```python
from build123d import *

# Parameters (mm, degrees)
CROQUIS1_R              = 20
CROQUIS1_R_2            = 15
SALIENTE_EXTRUIR1_DEPTH = 10
CROQUIS2_R              = 20
SALIENTE_EXTRUIR2_DEPTH = 2
CROQUIS3_R              = 12.5
SALIENTE_EXTRUIR3_DEPTH = 30
CORTAR_EXTRUIR2_DEPTH   = 10


with BuildPart() as part:
    # Croquis1 → Saliente-Extruir1 (new body)
    with BuildSketch(Plane(origin=(0, 0, 0), x_dir=(1, 0, 0), z_dir=(0, 1, 0))):
        with Locations(Location((0, 0, 0), (0, 0, 270))):
            Circle(CROQUIS1_R)
        with Locations(Location((0, 0, 0), (0, 0, 270))):
            Circle(CROQUIS1_R_2, mode=Mode.SUBTRACT)
    extrude(amount=-SALIENTE_EXTRUIR1_DEPTH)

    # Croquis2 → Saliente-Extruir2 (add)
    with BuildSketch(Plane.XZ.offset(10)):
        with Locations(Location((0, 0, 0), (0, 0, 90))):
            Circle(CROQUIS2_R)
    extrude(amount=SALIENTE_EXTRUIR2_DEPTH)

    # Croquis3 → Saliente-Extruir3 (add)
    with BuildSketch(Plane.XZ.offset(12)):
        with Locations(Location((0, 0, 0), (0, 0, 270))):
            Circle(CROQUIS3_R)
    extrude(amount=SALIENTE_EXTRUIR3_DEPTH)

    # Croquis4 → Cortar-Extruir2 (cut, symmetric)
    with BuildSketch(Plane.XY):
        Polygon((-15.546090629, -15.510770255), (-15.546090629, -25.510770255), (14.453909371, -39.5), (14.453909371, -29.5), align=None)
    extrude(amount=CORTAR_EXTRUIR2_DEPTH, both=True, mode=Mode.SUBTRACT)


solid = part.part
```
Part model, mm, in its own coordinate system. A direction names the side the tool comes from. Round coordinates to 2 decimals unless told otherwise and drop trailing zeros. Write each loop counter-clockwise with the first axis right and the second up, starting at its lowest first coordinate (ties: lowest second). Pieces come first, ordered by that corner, then holes. Notation, with made-up numbers: M 10.5,56 L 30.5,56 A16 ccw 30.5,81 Z; hole C -36.5,51.5 d3. An arc over 180 degrees is marked long. One line per question, with ' | ' between items.
(1) Probe line 1 along X through (y, z) = (-7, 0); line 2 along Y through (x, z) = (6, 0.5); line 3 along Z through (x, y) = (0.5, -39). List the from-to ranges inside material, lowest first.
Answer key:
line 1: x = -20 to -15, 15 to 20 | line 2: y = -42 to -35.56, -25.56 to -10 | line 3: z = -12.49 to 12.49
(2) Saw through at C-C on x = -6. Write the cut outline in (y, z), then the cut area to 3 significant figures.
Answer key:
outline: M -42,-10.97 L -12,-10.97 L -12,-19.08 L 0,-19.08 L 0,-13.75 L -10,-13.75 L -10,13.75 L 0,13.75 L 0,19.08 L -12,19.08 L -12,10.97 L -42,10.97 Z; hole M -29.96,-10 L -19.96,-10 L -19.96,10 L -29.96,10 Z | area: 641 mm^2
(3) 3-axis set-ups, long thin cutter, end or side, ignore diameter. For faces 5 (the face through (0, -28, -10)), 6 (the face through (0.66, -4.93, -14.985)), 7 (the face through (19.524, -5.916, -4.336)), 8 (the face through (-9, -12, 9)): which of +Z, -Z, +X, -X, +Y, -Y reach the whole face in a straight line?
Answer key:
face 5: none | face 6: +Y | face 7: +Y, -Y | face 8: -Y
(4) Saw through at A-A on z = 0. Write the cut outline in (x, y), then the cut area to 3 significant figures.
Answer key:
outline: M -20,-12 L -12.5,-12 L -12.5,-16.93 L 12.5,-28.59 L 12.5,-12 L 20,-12 L 20,0 L 15,0 L 15,-10 L -15,-10 L -15,0 L -20,0 Z; M -12.5,-42 L 12.5,-42 L 12.5,-38.59 L -12.5,-26.93 Z | area: 680 mm^2
(5) Saw through at D-D on y = -34.5. Write the cut outline in (x, z), then the cut area to 3 significant figures.
Answer key:
outline: M 3.73,-10 L 3.73,10 L 7.5,10 A12.5 ccw long 7.5,-10 Z | area: 346 mm^2
(6) Saw through at B-B on x = 9. Write the cut outline in (y, z).
Answer key:
outline: M -42,-8.67 L -36.96,-8.67 L -36.96,8.67 L -42,8.67 Z; M -26.96,-8.67 L -12,-8.67 L -12,-17.86 L 0,-17.86 L 0,-12 L -10,-12 L -10,12 L 0,12 L 0,17.86 L -12,17.86 L -12,8.67 L -26.96,8.67 Z
(7) Pin check, flat tips, straight feed: pin 1 (2 mm diameter, centred on x = 9, z = -15, fed in from -Y); pin 2 (7.5 mm diameter, centred on x = 0, y = -25.5, fed in from -Z); pin 3 (7.5 mm diameter, centred on x = 3, y = -24.5, fed in from +Z). Stop position of each tip, or through.
Answer key:
pin 1: stops at y = -12 | pin 2: stops at z = -12.5 | pin 3: stops at z = 12.5
(8) Two-plate mould, pull along Z, no slides. Class faces 1 (the face through (0, -42, 0)), 2 (the face through (-4.788, -26.79, -11.547)), 3 (the face through (0, -28, 10)), 4 (the face through (0, -10, 0)): released by +Z, released by -Z, zero draft, split by the parting line, or undercut.
Answer key:
face 1: zero draft | face 2: split by the parting line | face 3: undercut | face 4: undercut
